Model file for the job. Use its own axes, mm. Face numbers are marked on the shaded views. A direction names the side the tool comes from. Coordinates: 2 decimals unless noted, no trailing zeros. Order: outer loops, then holes, each group sorted by start corner. A loop starts at its lowest first (then second) coordinate and runs counter-clockwise, first axis right, second up. Notation, with made-up numbers: (-6.5, 48.25) - (21.5, 48.25) arc R9 ccw to (21.5, 63.25) - close; hole circle Ø9 at (-10, 3). An arc over 180 degrees is marked (long way). Put each result on its own line as item: value. Start each with the question number.
```python
from build123d import *

# Parameters (mm, degrees)
F0_W     = 381
F0_H     = 254
F1_DEPTH = 50.8
F2_R     = 6.35
F3_R     = 5.08
F5_W     = 368.3
F5_H     = 241.3
F6_DEPTH = 50.8
F7_R     = 3.175


with BuildPart() as f1:
    # F0 (on Front) → F1 (new body)
    with BuildSketch(Plane.XZ):
        Rectangle(F0_W, F0_H)
    extrude(amount=F1_DEPTH)

    # F2
    f2_edges = [f1.edges().sort_by_distance(p)[0] for p in [
        (190.5, -25.4, 127),
    ]]
    fillet(f2_edges, radius=F2_R)

    # F3
    f3_edges = [f1.edges().sort_by_distance(p)[0] for p in [
        (190.5, -25.4, -127),
        (-190.5, -25.4, 127),
        (-190.5, -25.4, -127),
    ]]
    fillet(f3_edges, radius=F3_R)


with BuildPart() as f1_1:
    # F4: moved
    add(f1.part.moved(Location((0, 50.8, 0))))

    # F5 (on Front) → F6 (cut)
    with BuildSketch(Plane.XZ):
        Rectangle(F5_W, F5_H)
    extrude(amount=-F6_DEPTH, mode=Mode.SUBTRACT)

    # F7
    f7_edges = [f1_1.edges().sort_by_distance(p)[0] for p in [
        (-184.15, 25.4, -120.65),
        (-184.15, 25.4, 120.65),
        (184.15, 25.4, -120.65),
        (184.15, 25.4, 120.65),
    ]]
    fillet(f7_edges, radius=F7_R)


with BuildPart() as f1_2:
    # F8: moved
    add(f1_1.part.moved(Location((0, 50.8, 0))))


with BuildPart() as f1_3:
    # F9: moved
    add(f1_2.part.moved(Location((0, 203.2, 0))))


solid = f1_3.part
```
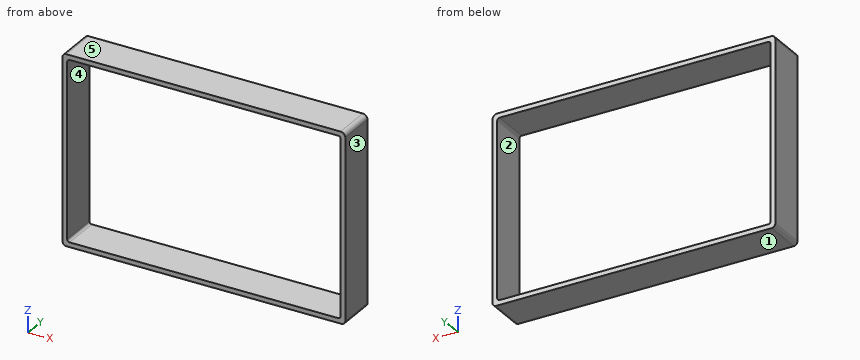
Item 1: Slice it at A-A, the plane y = 263. Give the cut face in (x, z) (3 decimals).
Item 2: Slice it at C-C, the plane z = 10. Give the cut face in (x, y), plus the area to 3 significant figures.
Item 3: 3-axis set-ups, long thin cutter, end or side, ignore diameter. For the marked faces 4 and 5: which of +Z, -Z, +X, -X, +Y, -Y reach the whole face in a straight line?
Item 4: Wall check: line 1 along X through (y, z) = (261.5, -107); line 2 along Z through (x, y) = (158, 259). Give the ranges that are in metal, low to high.
Item 5: Slice it at B-B, the plane x = 48. Give the cut face in (y, z), plus the area to 3 significant figures.
Item 6: Pull direction Z, two halves, no side cores. Call the marked faces 1, 2 and 3: pulls with the +Z half, pulls with the -Z half, needs draft (parallel to the pull), parting line crosses it, or undercut.
Here are the results:
1. outline: (-190.5, -121.92) arc R5.08 ccw to (-185.42, -127) - (185.42, -127) arc R5.08 ccw to (190.5, -121.92) - (190.5, 120.65) arc R6.35 ccw to (184.15, 127) - (-185.42, 127) arc R5.08 ccw to (-190.5, 121.92) - close; hole (-184.15, -117.475) arc R3.175 ccw to (-180.975, -120.65) - (180.975, -120.65) arc R3.175 ccw to (184.15, -117.475) - (184.15, 117.475) arc R3.175 ccw to (180.975, 120.65) - (-180.975, 120.65) arc R3.175 ccw to (-184.15, 117.475) - close
2. outline: (-190.5, 254) - (-184.15, 254) - (-184.15, 304.8) - (-190.5, 304.8) - close; (184.15, 254) - (190.5, 254) - (190.5, 304.8) - (184.15, 304.8) - close
2. area: 645 mm^2
3. face 4: +Y, -Y
3. face 5: +Z, +X, -X, +Y, -Y
4. line 1: x = -190.5 to -184.15, 184.15 to 190.5
4. line 2: z = -127 to -120.65, 120.65 to 127
5. outline: (254, -127) - (304.8, -127) - (304.8, -120.65) - (254, -120.65) - close; (254, 120.65) - (304.8, 120.65) - (304.8, 127) - (254, 127) - close
5. area: 645 mm^2
6. face 1: pulls with the -Z half
6. face 2: undercut
6. face 3: needs draft
